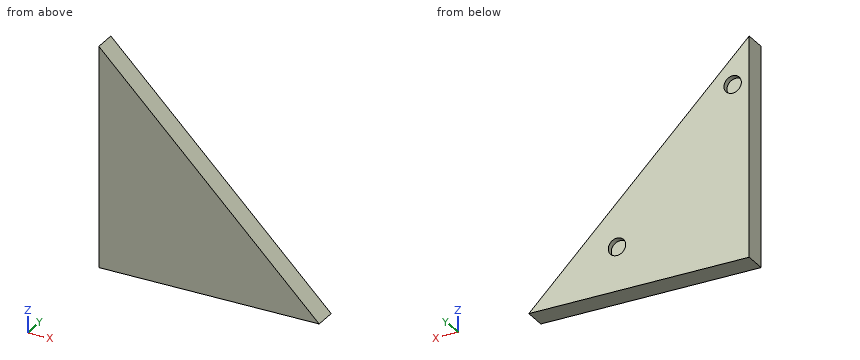
from build123d import *

# Parameters (mm, degrees)
F1_DEPTH = 25.4
F2_R     = 10.018842
F3_DEPTH = 6.35


with BuildPart() as f1:
    # F0 (on Front) → F1 (new body)
    with BuildSketch(Plane.XZ):
        Polygon((212.763246, -168.505661), (-41.236754, 85.494339), (-41.236754, -168.505661), align=None)
    extrude(amount=F1_DEPTH)

    # F2 (on face) → F3 (cut)
    with BuildSketch(Plane(origin=(0, 0, 0), x_dir=(-1, 0, 0), z_dir=(0, 1, 0))):
        with Locations((22.186754, 34.694339)):
            Circle(F2_R)
        with Locations((-111.163246, -117.705661)):
            Circle(F2_R)
    extrude(amount=-F3_DEPTH, mode=Mode.SUBTRACT)


solid = f1.part
Here's how the part is built. I have some questions about the finished solid (model axes, mm). Round coordinates to 2 decimals unless told otherwise and drop trailing zeros. Write each loop counter-clockwise with the first axis right and the second up, starting at its lowest first coordinate (ties: lowest second). Pieces come first, ordered by that corner, then holes.
1. Will these pins go through, and if not, where does the flat tip stop? pin 1 Ø10 at (x, z) = (-26, 32) entering from +Y; pin 2 Ø1.5 at (y, z) = (-21.5, -29.5) entering from +X; pin 3 Ø1 at (x, y) = (61.5, -20) entering from +Z.
2. I need wall thicknesses on L1, parallel to X at y = -4.75, z = -125; L2, parallel to Z at x = 200, y = -6.5; L3, parallel to Z at x = 107, y = -22. Which ranges of each line are inside material? Lowest first, please.
3. Suppose I cut it at B-B (x = 193). List the corners of the cut face in (y, z) for me.
4. Suppose I cut it at A-A (y = -15.75). List the corners of the cut face in (x, z) for me.
5. Suppose I cut it at C-C (z = -85.5). List the corners of the cut face in (x, y) for me.
Answer sheet:
1. pin 1: stops at y = -6.35
1. pin 2: stops at x = 74.51
1. pin 3: stops at z = -16.74
2. L1: x = -41.24 to 104.3, 118.03 to 169.26
2. L2: z = -168.51 to -155.74
2. L3: z = -168.51 to -62.74
3. outline: (-25.4, -168.51) - (0, -168.51) - (0, -148.74) - (-25.4, -148.74) - close
4. outline: (-41.24, -168.51) - (212.76, -168.51) - (-41.24, 85.49) - close
5. outline: (-41.24, -25.4) - (129.76, -25.4) - (129.76, 0) - (-41.24, 0) - close
